```python
from build123d import *

# Parameters (mm, degrees)
F1_DEPTH = 63.5
F2_DEPTH = 25.4
F3_DEPTH = 7.9375
F0_W     = 25.4
F0_H     = 19.05
F5_R     = 6.35


with BuildPart() as f1:
    # F0 (on Front) → F1 (new body, symmetric)
    with BuildSketch(Plane.XZ):
        Polygon((-41.275, 9.525), (-41.275, -9.525), (41.275, -9.525), (41.275, 9.525), (22.225, 9.525), align=None)
    extrude(amount=F1_DEPTH, both=True)

    # F0 (on Front) → F2 (join, symmetric)
    with BuildSketch(Plane.XZ):
        with BuildLine():
            Line((22.225, 9.525), (41.275, 9.525))
            Line((41.275, 9.525), (41.275, 27.0002))
            ThreePointArc((41.275, 27.0002), (45.9246798487, 38.2255201513), (57.15, 42.8752))
            Line((57.15, 42.8752), (60.325, 42.8752))
            Line((60.325, 42.8752), (60.325, 61.9252))
            Line((60.325, 61.9252), (57.15, 61.9252))
            add(Edge.make_bspline(
                [(55.5876742253, 61.8902381653), (56.1088932131, 61.9027160725), (56.6296931804, 61.9143561764), (57.15, 61.9252)],
                knots=[110.264215812, 110.264215812, 110.264215812, 110.264215812, 111.5045361635, 111.5045361635, 111.5045361635, 111.5045361635], degree=3))
            ThreePointArc((55.5876742253, 61.8902381653), (31.9079730144, 51.137219258), (22.225, 27.0002))
            Line((22.225, 27.0002), (22.225, 9.525))
        make_face()
    extrude(amount=F2_DEPTH, both=True)

    # F0 (on Front) → F3 (join, symmetric)
    with BuildSketch(Plane.XZ):
        with BuildLine():
            add(Edge.make_bspline(
                [(-41.275, 9.525), (-40.3964327978, 53.0503686598), (9.2514169059, 60.7809548666), (55.5876742253, 61.8902381653)],
                knots=[0, 0, 0, 0, 110.264215812, 110.264215812, 110.264215812, 110.264215812], degree=3))
            Line((-41.275, 9.525), (22.225, 9.525))
            Line((22.225, 9.525), (22.225, 27.0002))
            ThreePointArc((22.225, 27.0002), (31.9079730144, 51.137219258), (55.5876742253, 61.8902381653))
        make_face()
    extrude(amount=F3_DEPTH, both=True)

    # F0 (on Front) → F4 (revolve)
    with BuildSketch(Plane.XZ):
        with Locations((73.025, 52.4002)):
            Rectangle(F0_W, F0_H)
    revolve(axis=Axis((60.325, 0, 52.3875), (0, 0, 1)))

    # F5
    f5_edges = [f1.edges().sort_by_distance(p)[0] for p in [
        (-41.275, -63.5, 0),
        (41.275, -63.5, 0),
        (41.275, 63.5, 0),
        (-41.275, 63.5, 0),
    ]]
    fillet(f5_edges, radius=F5_R)


solid = f1.part
```
CAD build for the part. Positions are in the model's coordinates, mm. A direction names the side the tool comes from. Coordinates: 2 decimals unless noted, no trailing zeros. Order: outer loops, then holes, each group sorted by start corner. A loop starts at its lowest first (then second) coordinate and runs counter-clockwise, first axis right, second up. Notation, with made-up numbers: (42.25, 17) -> (70.25, 17) arc R18 cw to (70.25, 46) -> close; hole circle Ø8 at (49, 19). An arc over 180 degrees is marked (long way). Use one line per item in the form item = value. Start each with the question number.
1) Band-saw the part on B-B on y = -34. Give the cut face in (x, z) (3 decimals), then the cut area to 3 significant figures.
2) Band-saw the part on A-A on z = 1. Give the cut face in (x, y) (3 decimals), then the cut area to 3 significant figures.
3) Tool access for faces 1 (the cylindrical face through (28.407, 16.547, 46.84)), 2 (the cylindrical face through (34.926, 0.171, 61.554)), 3 (the flat face through (37, 25.4, 36)), 4 (the flat face through (41.275, -1, 4)), 5 (the flat face through (-2, -7.938, 30)): list every direction of +Z, -Z, +X, -X, +Y, -Y with a clear straight run to the whole face (end or side of a thin tool).
4) Drill centre lines: L1, parallel to Y at x = -31, z = 14; L2, parallel to Y at x = 35, z = 15; L3, parallel to Z at x = 0, y = 10.5 (3 decimals). Where is each one in solid material? Low to high. Write a range as [from, to].
5) Drop flat-ended pins along their axis: pin 1 (8.5 mm diameter, centred on y = 18.5, z = 15, fed in from -X) (3 decimals); pin 2 (12 mm diameter, centred on x = 22, z = 41.5, fed in from +Y); pin 3 (10 mm diameter, centred on y = 23, z = 52, fed in from -X); pin 4 (1.5 mm diameter, centred on y = -45, z = 11.5, fed in from -X). Give the stop position or say it passes through.
Entries:
q1.outline = (-41.275, -9.525) -> (41.275, -9.525) -> (41.275, 9.525) -> (-41.275, 9.525) -> close
q1.area = 1,570 mm2
q2.outline = (-41.275, -57.15) arc R6.35 ccw to (-34.925, -63.5) -> (34.925, -63.5) arc R6.35 ccw to (41.275, -57.15) -> (41.275, 57.15) arc R6.35 ccw to (34.925, 63.5) -> (-34.925, 63.5) arc R6.35 ccw to (-41.275, 57.15) -> close
q2.area = 10,400 mm2
q3.face_1 = +Z, -X, +Y
q3.face_2 = +Z, -X
q3.face_3 = +Z, +X, -X, +Y
q3.face_4 = -Z, +X, +Y, -Y
q3.face_5 = +Z, -X, -Y
q4.L1 = [-7.94, 7.94]
q4.L2 = [-25.4, 25.4]
q4.L3 = [-9.525, 9.525]
q5.pin_1 = 22.225
q5.pin_2 = 25.4
q5.pin_3 = 28.52
q5.pin_4 = through
